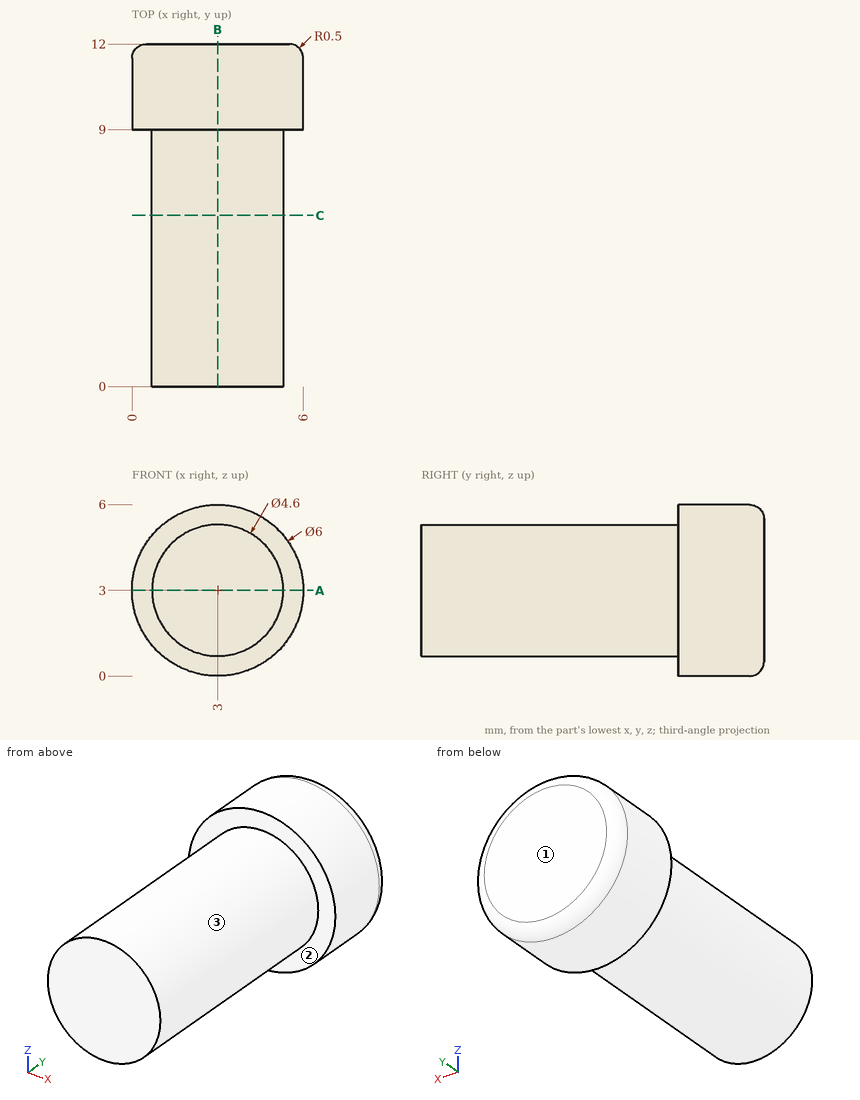
Study the drawing (mm; zero at the part's minimum x, y, z) and answer. Coordinates: 2 decimals unless noted, no trailing zeros. Order: outer loops, then holes, each group sorted by start corner. A loop starts at its lowest first (then second) coordinate and runs counter-clockwise, first axis right, second up. Notation, with made-up numbers: M 44,78 L 83,78 A24 ccw 83,88 Z; hole C -26.5,-11.5 d11. An arc over 180 degrees is marked long. Answer as a JSON object with one key per item and string values. Group by question number.
1. Straight lines are drawn through the part: line 1 (Y direction, x = 5.45, z = 3.6); line 2 (Y direction, x = 1.15, z = 1); line 3 (Z direction, x = 3.3, y = 3.75). For each, find the intervals that lie inside material, in ascending order.
2. Flat-ended cylindrical pins translate along their axes: P1, Ø3, axis at y = 3.5, z = 1.5, coming from the -X side; P2, Ø1.5, axis at x = 5, y = 10, coming from the +Z side; P3, Ø1.5, axis at x = 4, y = 9, coming from the -Z side. Find the tip coordinate at first contact, or state that the pin passes through.
3. Section A-A on z = 3 is taken. Write down the section's boundary in (x, y).
4. Section B-B on x = 3 is taken. Write down the section's boundary in (y, z).
5. Determine the mould class of the marked faces 1, 2 and 3 for opening direction Y: released by +Y, released by -Y, zero draft, split by the parting line, or undercut.
6. Section C-C on y = 6 is taken. Write down the section's boundary in (x, z), then the cut area to 3 significant figures.
Values follow:
{
 "1": {"line 1": "9 to 12", "line 2": "9 to 11.95", "line 3": "0.72 to 5.28"},
 "2": {"P1": "x = 0.7", "P2": "z = 5.73", "P3": "z = 0.01"},
 "3": {"outline": "M 0,9 L 0.7,9 L 0.7,0 L 5.3,0 L 5.3,9 L 6,9 L 6,11.5 A0.5 ccw 5.5,12 L 0.5,12 A0.5 ccw 0,11.5 Z"},
 "4": {"outline": "M 0,0.7 L 9,0.7 L 9,0 L 11.5,0 A0.5 ccw 12,0.5 L 12,5.5 A0.5 ccw 11.5,6 L 9,6 L 9,5.3 L 0,5.3 Z"},
 "5": {"face 1": "released by +Y", "face 2": "released by -Y", "face 3": "zero draft"},
 "6": {"outline": "C 3,3 d4.6", "area": "16.6 mm2"}
}
